Input: part model. Units: mm. Frame: model coordinates. A direction names the side the tool comes from. Round coordinates to 2 decimals unless told otherwise and drop trailing zeros. Order: outer loops, then holes, each group sorted by start corner. A loop starts at its lowest first (then second) coordinate and runs counter-clockwise, first axis right, second up. Notation, with made-up numbers: M 42,-29.75 L 84,-29.75 A22 ccw 84,-17.75 Z; hole C 4.5,10.25 d10. An arc over 180 degrees is marked long. One line per question, with ' | ' between items.
```python
from build123d import *

# Parameters (mm, degrees)
SKETCH1_R           = 2
BOSS_EXTRUDE1_DEPTH = 4
BOSS_EXTRUDE2_START = 3.1
SKETCH2_R           = 2
BOSS_EXTRUDE2_DEPTH = 3.1
BOSS_EXTRUDE3_DEPTH = 5


with BuildPart() as part:
    # Sketch1 → Boss-Extrude1 (new body)
    with BuildSketch(Plane.XY):
        with BuildLine():
            Line((-44, 0), (-44, 9))
            ThreePointArc((-44, 9), (-41.171572875, 10.171572875), (-40, 13))
            ThreePointArc((-40, 13), (-38.828427125, 15.828427125), (-36, 17))
            Line((-36, 17), (-32, 17))
            Line((-32, 17), (-32, 0))
            Line((-32, 0), (-44, 0))
        make_face()
        with Locations((-36, 13)):
            Circle(SKETCH1_R, mode=Mode.SUBTRACT)
    extrude(amount=BOSS_EXTRUDE1_DEPTH)

    # Sketch2 → Boss-Extrude2 (add)
    with BuildSketch(Plane(origin=(0, 0, 0), x_dir=(-1, 0, 0), z_dir=(0, 0, -1)).offset(BOSS_EXTRUDE2_START)):
        with BuildLine():
            Line((35, 9.3), (42.480131585, 9.3))
            ThreePointArc((42.480131585, 9.3), (40.677390057, 10.772835172), (40, 13))
            ThreePointArc((40, 13), (38.828427125, 15.828427125), (36, 17))
            Line((36, 17), (32.3, 17))
            Line((32.3, 17), (32.3, 12))
            ThreePointArc((32.3, 12), (33.090811691, 10.090811691), (35, 9.3))
        make_face()
        with Locations(Location((36, 13, 0), (0, 0, 180))):
            Circle(SKETCH2_R, mode=Mode.SUBTRACT)
    extrude(amount=-BOSS_EXTRUDE2_DEPTH)

    # Sketch4 → Boss-Extrude3 (add)
    with BuildSketch(Plane(origin=(-44, -0.024459729, 0), x_dir=(0, 0, 1), z_dir=(1, 0, 0))):
        Polygon((0.3, -11.324459729), (11, -22.024459729), (37, -22.024459729), (37, -0.024459729), (0, -0.024459729), (0, -9.324459729), (-3.1, -9.324459729), (-3.1, -11.324459729), align=None)
    extrude(amount=BOSS_EXTRUDE3_DEPTH)

    # Mirror1: part across plane


with BuildPart() as part_1:
    add(part.part)
    add(part.part.mirror(Plane(origin=(-44, 0, 4), x_dir=(0, 0, 1), z_dir=(0, 1, 0))))


solid = part_1.part
```
Item 1: Section query C-C, the plane y = 2.5. Return loops of the section in (x, z), plus the area to 3 significant figures.
Report:
outline: M -44,0 L -32,0 L -32,4 L -39,4 L -39,37 L -44,37 Z | area: 213 mm²
Item 2: Section query B-B, the plane x = -34.5. Return loops of the section in (y, z), plus the area to 3 significant figures.
Report:
outline: M -17,-3.1 L -14.32,-3.1 L -14.32,4 L -17,4 Z; M -11.68,-3.1 L -9.35,-3.1 L -9.35,0 L 9.35,0 L 9.35,-3.1 L 11.68,-3.1 L 11.68,4 L -11.68,4 Z; M 14.32,-3.1 L 17,-3.1 L 17,4 L 14.32,4 Z | area: 146 mm²
Item 3: Line query: line 1 along Y through (x, z) = (-36, -1); line 2 along X through (y, z) = (13, -1); line 3 along Y through (x, z) = (-36, 0.5). Output: solid intervals per line, ascending. Write a range as from..to.
Report:
line 1: -17..-15, -11..-9.3, 9.3..11, 15..17 | line 2: -40..-38, -34..-32.3 | line 3: -17..-15, -11..11, 15..17
Item 4: First-contact query: pin 1 (2 mm diameter, centred on y = -8.5, z = 29, fed in from +X); pin 2 (1.6 mm diameter, centred on x = -39.5, z = -1.5, fed in from +Y); pin 3 (2.5 mm diameter, centred on x = -42, z = -1, fed in from +Y); pin 4 (3.5 mm diameter, centred on x = -36, y = 13, fed in from -Z). Flat tips, straight axial feed; report the tip coordinate or a pass-through.
Report:
pin 1: x = -39 | pin 2: y = 15.95 | pin 3: y = 11.3 | pin 4: through
Item 5: Section query D-D, the plane z = 24. Return loops of the section in (x, y).
Report:
outline: M -44,-22 L -39,-22 L -39,22 L -44,22 Z
Item 6: Access query for faces 4 (the flat face through (-42, -11.3, -1)), 5 (the flat face through (-32.3, -15, -2)), 6 (the cylindrical face through (-33.07, 10.11, -1.57)). Directions: +Z, -Z, +X, -X, +Y, -Y. A direction counts if a zero-diameter tool reaches every point of the face in a straight line with its end or side. Return the directions, or none.
Report:
face 4: -Z, -X, -Y | face 5: -Z, +X, +Y, -Y | face 6: -Z, +X
Item 7: Section query A-A, the plane z = -0.5. Return loops of the section in (x, y), plus the area to 3 significant figures.
Report:
outline: M -44,-11.3 L -40.38,-11.3 A4 cw -40,-13 A4 ccw -36,-17 L -32.3,-17 L -32.3,-12 A2.7 ccw -35,-9.3 L -44,-9.3 Z; M -44,9.3 L -35,9.3 A2.7 ccw -32.3,12 L -32.3,17 L -36,17 A4 ccw -40,13 A4 cw -40.38,11.3 L -44,11.3 Z; hole C -36,-13 d4; hole C -36,13 d4 | area: 99.9 mm²
Item 8: Mould query, pull axis Y, two halves, no side actions, for faces 1 (the flat face through (-42, -17, 6)), 2 (the flat face through (-38, -12, -3.1)), 3 (the flat face through (-40, -9.3, -2)). Classes: +Y half, -Y half, draft (parallel to the pull), parting line (faces both ways), or undercut.
Report:
face 1: -Y half | face 2: draft | face 3: undercut
